Autodesk Inventor part; units mm, degrees
ref_plane "YZ Plane" through (0, 0, 0) normal (1, 0, 0) x (0, 1, 0)
ref_plane "XZ Plane" through (0, 0, 0) normal (0, 1, 0) x (-1, 0, 0)
ref_plane "XY Plane" through (0, 0, 0) normal (0, 0, 1) x (1, 0, 0)
sketch "Sketch3" plane through (0, 0, 0) normal (0, 0, 1) x (1, 0, 0)
  circle A0 centre (51, -10.8228) radius 2
  circle A1 centre (33, -10.8228) radius 2
  circle A2 centre (15, -10.8228) radius 2
  line L0 (0, -18.3228) -> (60, -18.3228)
  line L1 (0, -18.3228) -> (0, -13.3228)
  line L2 (10, -13.3228) -> (0, -13.3228)
  line L3 (10, -3.3228) -> (10, -13.3228)
  line L4 (10, -3.3228) -> (57, -3.3228)
  line L5 (60, -18.3228) -> (60, -10.8228)
  circle A3 centre (-5, 77.6772) radius 2
  circle A4 centre (-5, 59.6772) radius 2
  circle A5 centre (-5, 23.6772) radius 2
  circle A6 centre (-5, 5.6772) radius 2
  circle A7 centre (-5, 41.6772) radius 2
  line L6 (-10, -18.3228) -> (-10, 101.6772)
  line L7 (-10, 101.6772) -> (0, 101.6772)
  line L8 (0, 96.6772) -> (0, 101.6772)
  line L9 (0, 96.6772) -> (10, 96.6772)
  line L10 (10, -13.3228) -> (10, 96.6772)
  line L11 (0, -13.3228) -> (10, -13.3228)
  line L12 (0, -18.3228) -> (0, -13.3228)
  line L13 (-10, -18.3228) -> (0, -18.3228)
  circle A8 centre (51, 94.1772) radius 2
  circle A9 centre (33, 94.1772) radius 2
  circle A10 centre (15, 94.1772) radius 2
  line L14 (0, 101.6772) -> (60, 101.6772)
  line L15 (60, 94.1772) -> (60, 101.6772)
  line L16 (10, 86.6772) -> (57, 86.6772)
  line L17 (10, 96.6772) -> (10, 86.6772)
  line L18 (0, 96.6772) -> (10, 96.6772)
  line L19 (0, 101.6772) -> (0, 96.6772)
  line L20 (57, -10.8228) -> (60, -10.8228)
  line L21 (57, -3.3228) -> (57, -10.8228)
  line L22 (60, 94.1772) -> (57, 94.1772)
  line L23 (57, 94.1772) -> (57, 86.6772)
  line L24 (57, 86.6772) -> (57, -4.2516)
  point P0 (0, 0)
extrude "Extrusion2" add sketch "Sketch3" along normal blind 3
properties part number "КВ33.000.103 - Стенка тонкая"
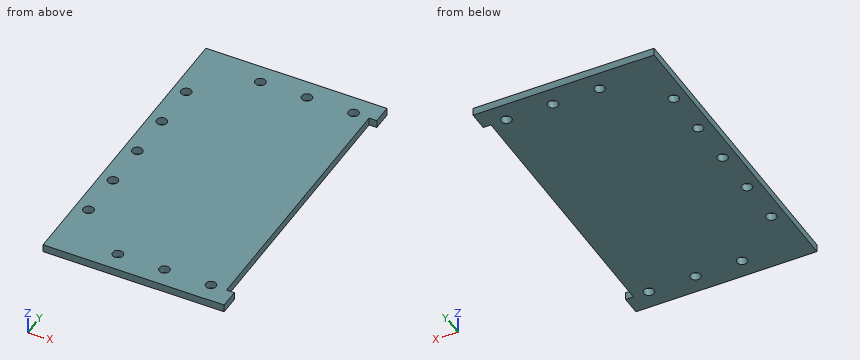
Work out the finished part from the listing and answer in its coordinate system (mm). Round coordinates to 2 decimals unless told otherwise and drop trailing zeros. Loops run counter-clockwise (first coordinate to the right, second up) from the corner with the lowest first, then second, coordinate; pieces in that order, holes last.
(1) The part is cut by section B-B, the plane x = -5. Give the vertices of the cut face in (y, z).
Computed values:
outline: (-18.32, 0) - (3.68, 0) - (3.68, 3) - (-18.32, 3) - close; (7.68, 0) - (21.68, 0) - (21.68, 3) - (7.68, 3) - close; (25.68, 0) - (39.68, 0) - (39.68, 3) - (25.68, 3) - close; (43.68, 0) - (57.68, 0) - (57.68, 3) - (43.68, 3) - close; (61.68, 0) - (75.68, 0) - (75.68, 3) - (61.68, 3) - close; (79.68, 0) - (101.68, 0) - (101.68, 3) - (79.68, 3) - close
(2) The part is cut by section D-D, the plane y = 1. Give the vertices of the cut face in (x, z).
Computed values:
outline: (-10, 0) - (57, 0) - (57, 3) - (-10, 3) - close
(3) The part is cut by section A-A, the plane x = 15. Give the vertices of the cut face in (y, z).
Computed values:
outline: (-18.32, 0) - (-12.82, 0) - (-12.82, 3) - (-18.32, 3) - close; (-8.82, 0) - (92.18, 0) - (92.18, 3) - (-8.82, 3) - close; (96.18, 0) - (101.68, 0) - (101.68, 3) - (96.18, 3) - close
(4) Find the intervals of material crossed by L1, parallel to Y at x = -5, z = 1.6; L2, parallel to Y at x = 33, z = 1.5; L3, parallel to Y at x = 50.5, z = 2.65, in increasing order.
Computed values:
L1: y = -18.32 to 3.68, 7.68 to 21.68, 25.68 to 39.68, 43.68 to 57.68, 61.68 to 75.68, 79.68 to 101.68
L2: y = -18.32 to -12.82, -8.82 to 92.18, 96.18 to 101.68
L3: y = -18.32 to -12.76, -8.89 to 92.24, 96.11 to 101.68
(5) The part is cut by section C-C, the plane z = 2.5. Give the number of separate pieces and of enclosed holes in the cut face, and give its area (3 significant figures).
Computed values:
separate pieces: 1
enclosed holes: 11
area: 7,950 mm2
(6) This flat-tipped pin is pushed along its axis until it touches: P1, Ø1, axis at y = 1.5, z = 0.5, coming from the +X side. Where does it stop, or does it pass through?
Computed values:
P1: stops at x = 57
